Check sheet for the drawn part. Datum: minimum x, y, z corner. Units: mm. A direction names the side the tool comes from. Coordinates: 2 decimals unless noted, no trailing zeros. Order: outer loops, then holes, each group sorted by start corner. A loop starts at its lowest first (then second) coordinate and runs counter-clockwise, first axis right, second up. Notation, with made-up numbers: M 35.5,-25 L 80.5,-25 A12 cw 80.5,-6 Z; hole C 14,-39 d1. An arc over 180 degrees is marked long. Answer in a Markdown table with one row per item. Add a question column.
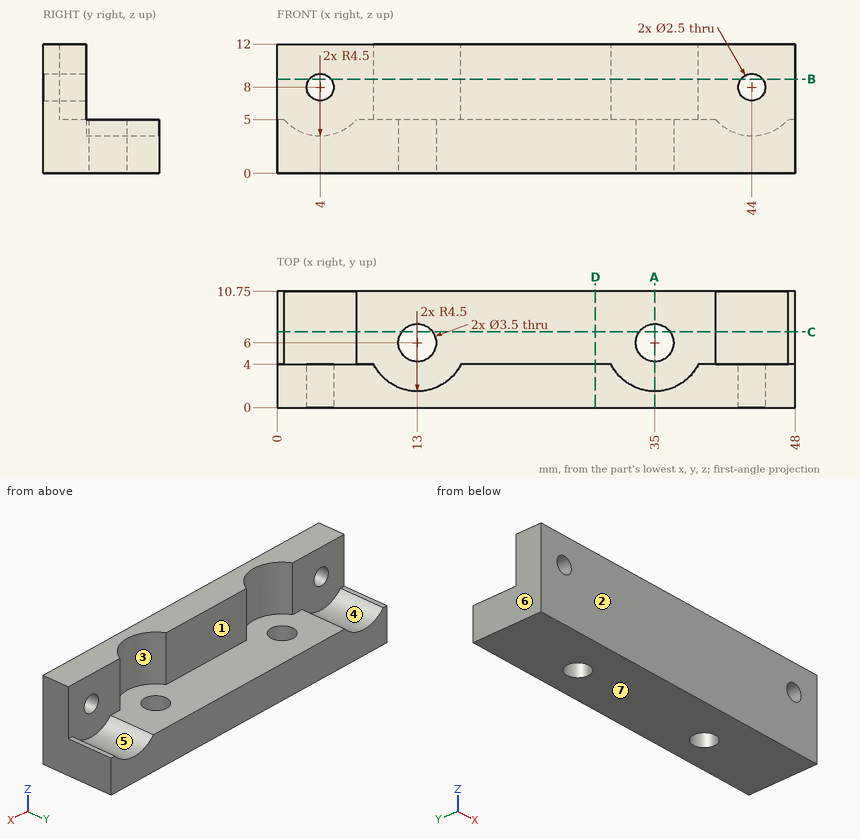
1. Section check C-C on y = 7. Enter the section's corners in (x, z).
2. Section check A-A on x = 35. Enter the section's corners in (y, z).
3. Section check D-D on x = 29.5. Enter the section's corners in (y, z), then the cut area to 4 significant figures.
4. Section check B-B on z = 8.75. Enter the section's corners in (x, y), then the cut area to 3 significant figures.
5. Go/stop test with flat-tipped pins: pin 1 Ø0.5 at (x, y) = (47.5, 8.5) entering from +Z; pin 2 Ø3.5 at (x, z) = (21.5, 8) entering from +Y. Record where each tip stops, or that it passes through.
6. Set-up check for the marked faces 1, 2 and 3: record each of +Z, -Z, +X, -X, +Y, -Y from which the full face is reachable in a straight line by a thin tool's end or side.
7. Release check for a two-part mould opening along X. For the marked faces 4, 5, 6 and 7 record: released by +X, released by -X, zero draft, split by the parting line, or undercut.
8. Scan lines: line 1 (X direction, y = 7, z = 4); line 2 (Z direction, x = 4, y = 1.9); line 3 (X direction, y = 9, z = 4.75). Record each from-to range of solid material in increasing order.
Result sheet:
| question | item | result |
|---|---|---|
| 1 | outline | M 0,0 L 11.56,0 L 11.56,5 L 7.35,5 A4.5 cw 0.65,5 L 0,5 Z; M 14.44,0 L 33.56,0 L 33.56,5 L 14.44,5 Z; M 36.44,0 L 48,0 L 48,5 L 47.35,5 A4.5 cw 40.65,5 L 36.44,5 Z |
| 2 | outline | M 0,0 L 4.25,0 L 4.25,5 L 1.5,5 L 1.5,12 L 0,12 Z; M 7.75,0 L 10.75,0 L 10.75,5 L 7.75,5 Z |
| 3 | outline | M 0,0 L 10.75,0 L 10.75,5 L 4,5 L 4,12 L 0,12 Z |
| 3 | area | 81.75 mm^2 |
| 4 | outline | M 0,0 L 3,0 L 3,4 L 0,4 Z; M 5,0 L 43,0 L 43,4 L 39.03,4 A4.5 cw 30.97,4 L 17.03,4 A4.5 cw 8.97,4 L 5,4 Z; M 45,0 L 48,0 L 48,4 L 45,4 Z |
| 4 | area | 147 mm^2 |
| 5 | pin 1 | z = 5 |
| 5 | pin 2 | y = 4 |
| 6 | face 1 | +Z, +X, -X, +Y |
| 6 | face 2 | +Z, -Z, +X, -X, -Y |
| 6 | face 3 | +Z, +Y |
| 7 | face 4 | undercut |
| 7 | face 5 | undercut |
| 7 | face 6 | released by -X |
| 7 | face 7 | zero draft |
| 8 | line 1 | 0 to 1.94, 6.06 to 11.56, 14.44 to 33.56, 36.44 to 41.94, 46.06 to 48 |
| 8 | line 2 | 0 to 6.75, 9.25 to 12 |
| 8 | line 3 | 0 to 0.89, 7.11 to 40.89, 47.11 to 48 |
